```python
from build123d import *

# Parameters (mm, degrees)
ESQUISSE1_R        = 12.5
ESQUISSE1_W        = 50
ESQUISSE1_H        = 50
BOSS_EXTRU_1_DEPTH = 5


with BuildPart() as part:
    # Esquisse1 → Boss.-Extru.1 (new body)
    with BuildSketch(Plane.XY):
        Polygon((-28.909774436, 20), (-23.909774436, 20), (-23.909774436, 15), (1.090225564, 15), (1.090225564, 20), (36.090225564, 20), (36.090225564, 15), (106.090225564, 15), (106.090225564, 20), (141.090225564, 20), (141.090225564, 15), (166.090225564, 15), (166.090225564, 20), (171.090225564, 20), (171.090225564, 5.001724715), (166.090225564, 5.001724715), (166.090225564, -14.998275285), (171.090225564, -14.998275285), (171.090225564, -44.998275285), (166.090225564, -44.998275285), (166.090225564, -64.998275285), (171.090225564, -64.998275285), (171.090225564, -79.99655057), (166.090225564, -79.99655057), (166.090225564, -74.99655057), (141.090225564, -74.99655057), (141.090225564, -79.99655057), (106.090225564, -79.99655057), (106.090225564, -74.99655057), (36.090225564, -74.99655057), (36.090225564, -79.99655057), (1.090225564, -79.99655057), (1.090225564, -74.99655057), (-23.909774436, -74.99655057), (-23.909774436, -79.99655057), (-28.909774436, -79.99655057), (-28.909774436, -64.998275285), (-23.909774436, -64.998275285), (-23.909774436, -59.99655057), (-23.909774436, -44.998275285), (-28.909774436, -44.998275285), (-28.909774436, -14.998275285), (-23.909774436, -14.998275285), (-23.909774436, 5), (-28.909774436, 5), align=None)
        with Locations((120, -29.998275285)):
            Circle(ESQUISSE1_R, mode=Mode.SUBTRACT)
        with Locations((25, -29.998275285)):
            Rectangle(ESQUISSE1_W, ESQUISSE1_H, mode=Mode.SUBTRACT)
    extrude(amount=BOSS_EXTRU_1_DEPTH)


solid = part.part
```
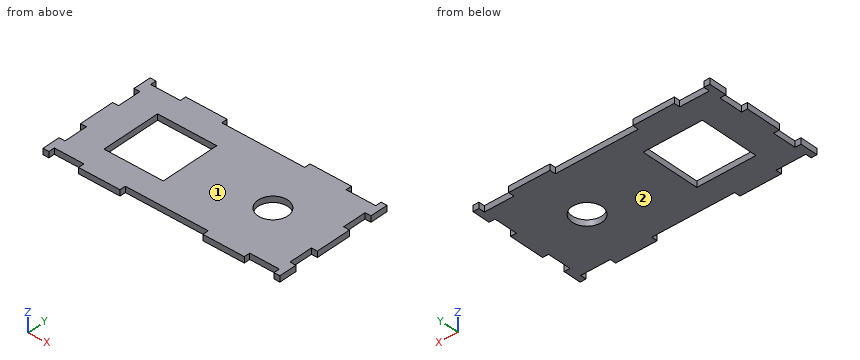
Read the model definition and answer for the solid it produces. Units are mm, in the model's axes. Face numbers are marked on the shaded views. Give positions to 0.01 mm unless a question says otherwise; leave off trailing zeros. Write each loop counter-clockwise with the first axis right and the second up, starting at its lowest first coordinate (ties: lowest second). Pieces come first, ordered by that corner, then holes. Notation, with made-up numbers: M 48,18.5 L 102,18.5 A15 cw 102,44.5 Z; hole C 61.5,1.5 d11. An arc over 180 degrees is marked long. Put each result on its own line as item: value. Start each with the question number.
1. The part is cut by section D-D, the plane z = 3.85. Give the number of separate pieces and of enclosed holes in the cut face, and give its area (3 significant figures).
2. The part is cut by section C-C, the plane y = -26. Give the vertices of the cut face in (x, z), and give its area (3 significant figures).
3. For a pull along Z with two mould halves and no side action, classify the marked faces 1 and 2 as released by +Z, released by -Z, zero draft, split by the parting line, or undercut.
4. The part is cut by section A-A, the plane y = -11. Give the vertices of the cut face in (x, z).
5. Consider line 1 along Y through (x, z) = (120, 3.5); line 2 along X through (y, z) = (-50, 0.4); line 3 along X through (y, z) = (-27.5, 3.3). Determine where each line is inside the solid, lowest interval first.
6. The part is cut by section B-B, the plane x = 120. Give the vertices of the cut face in (y, z).
Final values:
1. separate pieces: 1
1. enclosed holes: 2
1. area: 15,400 mm²
2. outline: M -28.91,0 L 0,0 L 0,5 L -28.91,5 Z; M 50,0 L 108.16,0 L 108.16,5 L 50,5 Z; M 131.84,0 L 171.09,0 L 171.09,5 L 131.84,5 Z
2. area: 632 mm²
3. face 1: released by +Z
3. face 2: released by -Z
4. outline: M -23.91,0 L 0,0 L 0,5 L -23.91,5 Z; M 50,0 L 166.09,0 L 166.09,5 L 50,5 Z
5. line 1: y = -80 to -42.5, -17.5 to 20
5. line 2: x = -23.91 to 0, 50 to 166.09
5. line 3: x = -28.91 to 0, 50 to 107.75, 132.25 to 171.09
6. outline: M -80,0 L -42.5,0 L -42.5,5 L -80,5 Z; M -17.5,0 L 20,0 L 20,5 L -17.5,5 Z
